Autodesk Inventor part; units mm, degrees
ref_plane "YZ Plane" through (0, 0, 0) normal (1, 0, 0) x (0, 1, 0)
ref_plane "XZ Plane" through (0, 0, 0) normal (0, 1, 0) x (-1, 0, 0)
ref_plane "XY Plane" through (0, 0, 0) normal (0, 0, 1) x (1, 0, 0)
sketch "Sketch1" plane through (0, 0, 0) normal (0, 0, 1) x (1, 0, 0)
  line L0 (0, 0) -> (80, 0)
  line L1 (80, 0) -> (80, 23)
  line L2 (80, 23) -> (0, 23)
  line L3 (0, 23) -> (0, 0)
  dimension "d0" = 80
  dimension "d1" = 23
extrude "Extrusion1" add sketch "Sketch1" along normal blind 12
sketch "Sketch2" plane through (0, 0, 0) normal (-1, 0, 0) x (0, 0, 1)
  line L0 (0, 23) -> (0, 0)
  line L1 (0, 0) -> (12, 0)
  line L2 (12, 23) -> (7, 23)
  line L3 (7, 23) -> (7, 5)
  line L4 (7, 5) -> (12, 5)
  line L5 (12, 5) -> (12, 23)
  dimension "d4" = 7
  dimension "d5" = 5
extrude "Extrusion2" cut sketch "Sketch2" against normal blind 80
sketch "Sketch3" plane through (0, 5, 7) normal (0, 0, 1) x (1, 0, 0)
  line L0 (0, 18) -> (80, 18)
  line L1 (0, 0) -> (0, 18)
  point P0 (0, -5)
  point P1 (22.5, 10.5)
  point P2 (57.5, 10.5)
  dimension "d8" = 7.5
  dimension "d9" = 7.5
  dimension "d10" = 35
  dimension "d11" = 22.5
hole "Hole1" at (22.5, 15.5, 7) at (57.5, 15.5, 7) direction (0, 0, -1) diameter 6.5 depth 7 tip angle 118 countersink diameter 11.5 countersink angle 90
fillet "Fillet1" radius 7 2 edges at (0, 14, 7) (80, 14, 7)
fillet "Fillet2" radius 5 2 edges at (0, 2.5, 12) (80, 2.5, 12)
properties part number "PÁRA-CHOQUE DIANTEIRO" material "Carbon Steel"
Work out the finished part from the listing and answer in its coordinate system (mm). A direction names the side the tool comes from. Give positions to 0.01 mm unless a question says otherwise; leave off trailing zeros. Write each loop counter-clockwise with the first axis right and the second up, starting at its lowest first coordinate (ties: lowest second). Pieces come first, ordered by that corner, then holes.
(1) Flat-ended cylindrical pins translate along their axes: pin 1 Ø2 at (y, z) = (8, 1.5) entering from +X; pin 2 Ø10 at (x, y) = (25, 14) entering from +Z; pin 3 Ø2 at (y, z) = (11, 6.5) entering from -X. Find the tip coordinate at first contact, or state that the pin passes through.
Final values:
pin 1: stops at x = 79.98
pin 2: stops at z = 7
pin 3: stops at x = 2.67
(2) The part is cut by section A-A on x = 22.5. Write down the section's boundary in (y, z).
Final values:
outline: (0, 0) - (12.25, 0) - (12.25, 4.5) - (9.75, 7) - (5, 7) - (5, 12) - (0, 12) - close; (18.75, 0) - (23, 0) - (23, 7) - (21.25, 7) - (18.75, 4.5) - close
(3) The part is cut by section D-D on z = 9.5. Write down the section's boundary in (x, y).
Final values:
outline: (0.67, 0) - (79.33, 0) - (79.33, 5) - (0.67, 5) - close
(4) The mould has two halves that part along Y. Classify faces 1 (the flat face through (39, 5, 9)), 2 (the conical face through (24.802, 18.011, 4.656)), 3 (the flat face through (39, 12, 0)): pulls with the +Y half, pulls with the -Y half, needs draft (parallel to the pull), parting line crosses it, or undercut.
Final values:
face 1: pulls with the +Y half
face 2: undercut
face 3: needs draft
(5) Straight lines are drawn through the part: line 1 (X direction, y = 15.5, z = 3.65); line 2 (Y direction, x = 57.5, z = 3.35); line 3 (X direction, y = 15.5, z = 1.5). For each, find the intervals that lie inside material, in ascending order.
Final values:
line 1: x = 1.03 to 19.25, 25.75 to 54.25, 60.75 to 78.97
line 2: y = 0 to 12.25, 18.75 to 23
line 3: x = 0.16 to 19.25, 25.75 to 54.25, 60.75 to 79.84
(6) The part is cut by section C-C on x = 34.5. Write down the section's boundary in (y, z), plus the area to 3 significant figures.
Final values:
outline: (0, 0) - (23, 0) - (23, 7) - (5, 7) - (5, 12) - (0, 12) - close
area: 186 mm2
(7) Which of the six approach directions +Z, -Z, +X, -X, +Y, -Y give full straight-line access (tool end or side, diameter ignored) to faces 4 (the cylindrical face through (78, 13.9, 4.9)), 5 (the flat face through (40, 14, 7)), 6 (the cylindrical face through (2.1, 13.9, 5))?
Final values:
face 4: +Z, +X, +Y
face 5: +Z, +X, -X, +Y
face 6: +Z, -X, +Y
(8) The part is cut by section B-B on y = 15.5. Count the separate pieces of the cut face and the enclosed holes in it, plus the area to 3 significant figures.
Final values:
separate pieces: 3
enclosed holes: 0
area: 435 mm2
